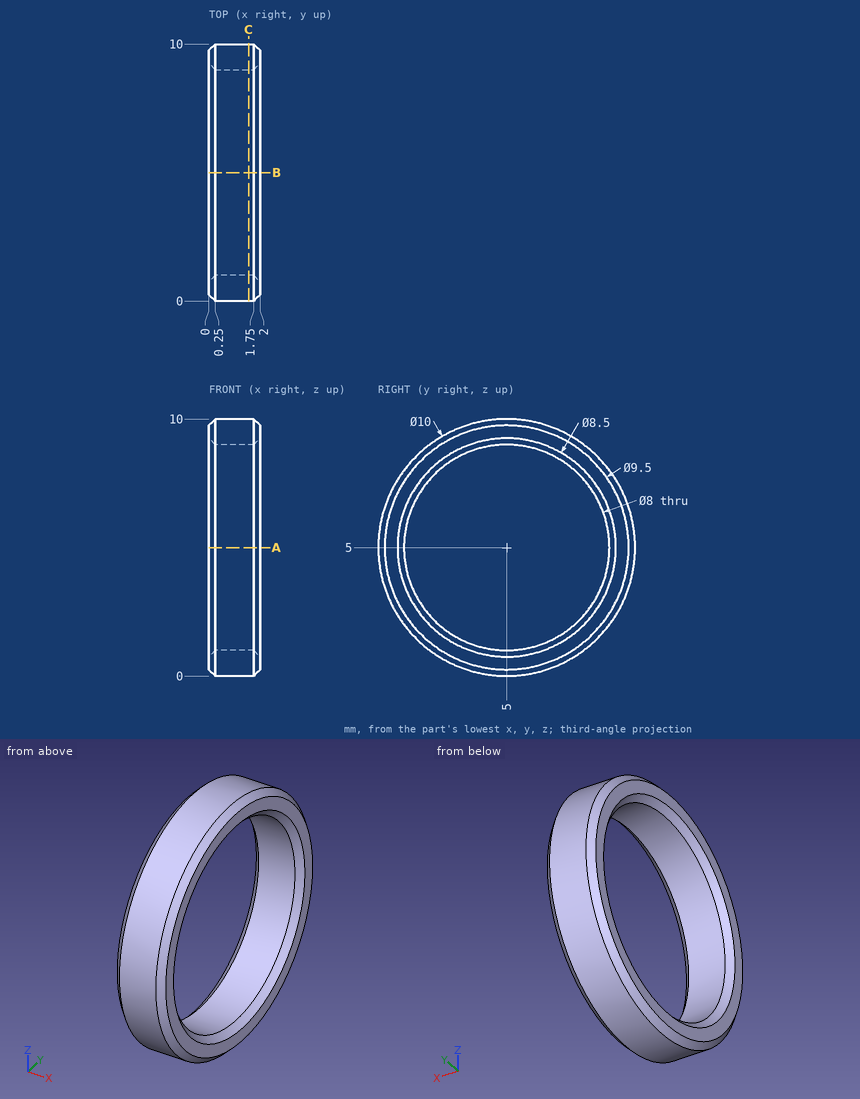
Geometry: see drawing. Coordinates: mm, zero at the bounding-box minimum. Coordinates: 2 decimals unless noted, no trailing zeros. Loops run counter-clockwise (first coordinate to the right, second up) from the corner with the lowest first, then second, coordinate; pieces in that order, holes last.
Q1. Cut plane C-C (x = 1.55). Output: boundary loops of the cut face in (y, z), then the cut area to 3 significant figures.
Q2. Contact query for a flat-ended pin moving along its axis: pin 1 (1 mm diameter, centred on x = 0, y = 8, fed in from -Z). Output: stop coordinate, or through.
Q3. Cut plane A-A (z = 5). Output: boundary loops of the cut face in (x, y).
Q4. Material intervals for line 1 (Z direction, x = 0.7, y = 5); line 2 (Z direction, x = 1.4, y = 4); line 3 (Y direction, x = 1.1, z = 7.5), sorted ascending.
Working result:
1. outline: circle Ø10 at (5, 5); hole circle Ø8 at (5, 5)
1. area: 28.3 mm2
2. pin 1: stops at z = 0.71
3. outline: (0, 0.25) - (0.25, 0) - (1.75, 0) - (2, 0.25) - (2, 0.75) - (1.75, 1) - (0.25, 1) - (0, 0.75) - close; (0, 9.25) - (0.25, 9) - (1.75, 9) - (2, 9.25) - (2, 9.75) - (1.75, 10) - (0.25, 10) - (0, 9.75) - close
4. line 1: z = 0 to 1, 9 to 10
4. line 2: z = 0.1 to 1.13, 8.87 to 9.9
4. line 3: y = 0.67 to 1.88, 8.12 to 9.33
